```python
from build123d import *

# Parameters (mm, degrees)
F1_DEPTH = 5
F3_DEPTH = 25


with BuildPart() as f1:
    # F0 (on Front) → F1 (new body)
    with BuildSketch(Plane.XZ):
        with BuildLine():
            Line((0, 20), (-120, 26))
            Line((-120, 26), (-120, 15))
            Line((-120, 15), (-110.250925, 12.773895))
            ThreePointArc((-110.250925, 12.773895), (-107.888962, 12.158173), (-105.568952, 11.399531))
            Line((-105.568952, 11.399531), (-87.172784, 4.756131))
            ThreePointArc((-87.172784, 4.756131), (-73.792942, 1.198003), (-60, 0))
            Line((-60, 0), (0, 0))
            Line((0, 0), (0, 20))
        make_face()
    extrude(amount=F1_DEPTH)

    # F2 (on face) → F3 (cut)
    with BuildSketch(Plane.XZ.offset(5)):
        Polygon((-6.242202, 15.305864), (-5.992514, 20.299626), (-30.961323, 21.548066), (-31.211011, 16.554304), align=None)
    extrude(amount=-F3_DEPTH, mode=Mode.SUBTRACT)


solid = f1.part
```
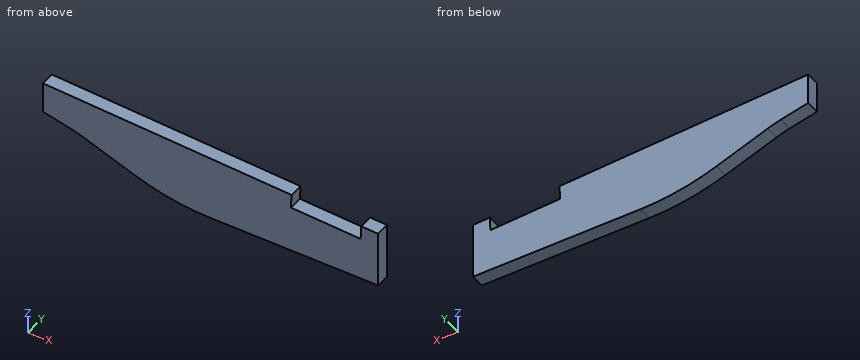
The listing builds one solid part. Answer for the finished solid, in the listing's coordinates (mm). Give positions to 0.01 mm unless a question says otherwise; leave off trailing zeros. Write each loop counter-clockwise with the first axis right and the second up, starting at its lowest first coordinate (ties: lowest second). Pieces come first, ordered by that corner, then holes. Notation, with made-up numbers: (44.5, -32.75) -> (53.5, -32.75) arc R20 ccw to (53.5, -15.75) -> close; hole circle Ø7 at (41, 17). An arc over 180 degrees is marked (long way). Use one line per item in the form item = value.
1) Straight lines are drawn through the part: probe 1 along X at (y, z) = (-2.55, 17.25) (3 decimals); probe 2 along Z at (x, y) = (-83, -4.3); probe 3 along Z at (x, y) = (-27, -4.25). For each, find the intervals that lie inside material, in ascending order.
Result:
probe_1 = -120 to -31.176, -6.145 to 0
probe_2 = 3.38 to 24.15
probe_3 = 0 to 16.34
2) Section B-B on z = 18 is taken. Write down the section's boundary in (x, y), plus the area to 3 significant figures.
Result:
outline = (-120, -5) -> (-31.14, -5) -> (-31.14, 0) -> (-120, 0) -> close; (-6.11, -5) -> (0, -5) -> (0, 0) -> (-6.11, 0) -> close
area = 475 mm²
3) Each of these flat-tipped pins is pushed along its axis until it touches: P1, Ø1.5, axis at x = -67, y = -3.5, coming from the -Z side; P2, Ø1, axis at x = -23, y = -0.5, coming from the -Z side; P3, Ø2, axis at x = -74, y = -2, coming from the +Z side. Where does it stop, or does it pass through?
Result:
P1 = 0.24
P2 = 0
P3 = 23.75
4) Section D-D on z = 23.5 is taken. Write down the section's boundary in (x, y).
Result:
outline = (-120, -5) -> (-70, -5) -> (-70, 0) -> (-120, 0) -> close
5) Section A-A on y = -0.8 is taken. Write down the section's boundary in (x, z), plus the area to 3 significant figures.
Result:
outline = (-120, 15) -> (-110.25, 12.77) arc R40 cw to (-105.57, 11.4) -> (-87.17, 4.76) arc R80 ccw to (-60, 0) -> (0, 0) -> (0, 20) -> (-5.99, 20.3) -> (-6.24, 15.31) -> (-31.21, 16.55) -> (-30.96, 21.55) -> (-120, 26) -> close
area = 2,250 mm²
6) Section C-C on x = -58 is taken. Write down the section's boundary in (y, z).
Result:
outline = (-5, 0) -> (0, 0) -> (0, 22.9) -> (-5, 22.9) -> close
